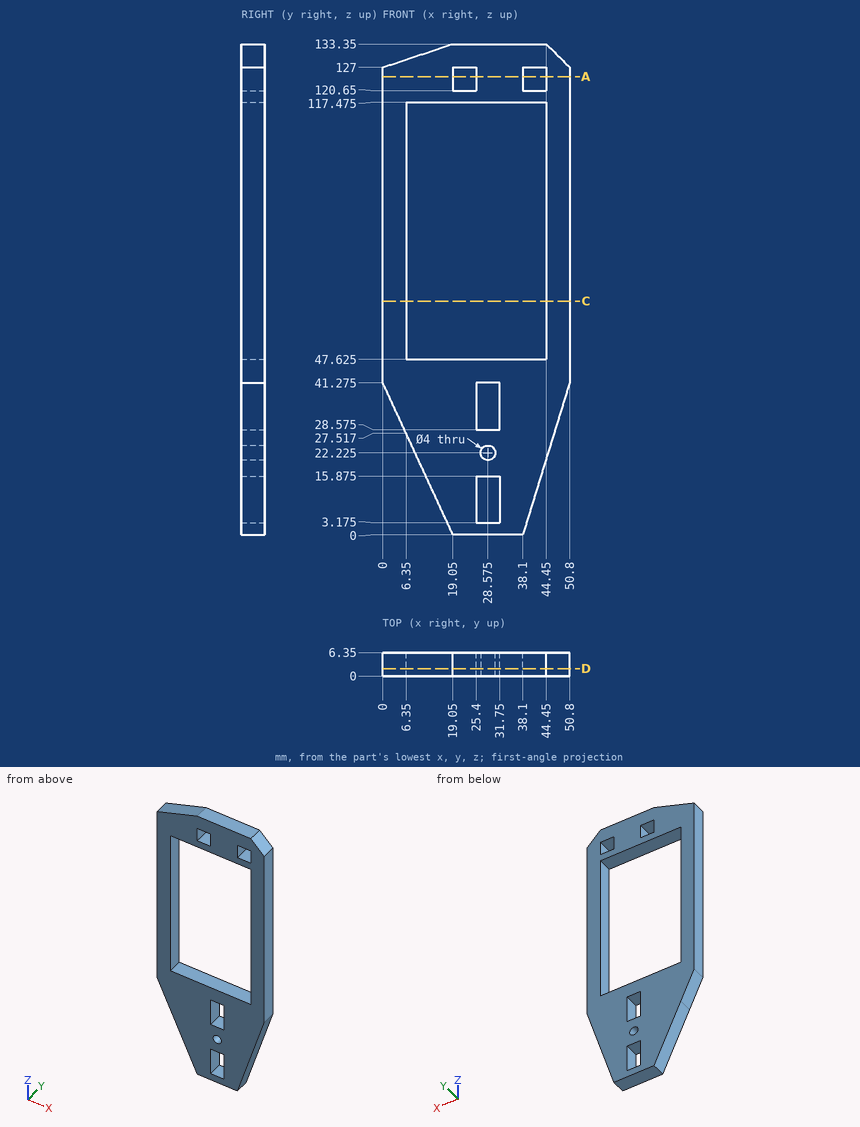
Geometry check sheet. Reference: drawing and pictorial views, mm from the part's lowest x, y, z. Give positions to 0.01 mm unless a question says otherwise; leave off trailing zeros. Order: outer loops, then holes, each group sorted by start corner. A loop starts at its lowest first (then second) coordinate and runs counter-clockwise, first axis right, second up. Notation, with made-up numbers: (44, 18) -> (60, 18) arc R22 cw to (60, 35) -> close; hole circle Ø1 at (88.5, 36). An arc over 180 degrees is marked (long way). Use CSV: the item, a comma, the result in double quotes. Start each with the question number.
1) Sectioned sample at A-A, the plane z = 124.5. Record the boundary of the cut face in (x, y).
2) Sectioned sample at C-C, the plane z = 63.5. Record the boundary of the cut face in (x, y).
3) Go/stop test with flat-tipped pins: P1, Ø3, axis at y = 4, z = 8, coming from the +X side; P2, Ø3, axis at y = 2.5, z = 36, coming from the -X side. Record where each tip stops, or that it passes through.
4) Sectioned sample at D-D, the plane y = 2. Give the number of separate pieces and of enclosed holes in the cut face, plus the area to 3 significant figures.
5) Material ranges on line 1 (X direction, y = 1.25, z = 51.5); line 2 (Z direction, x = 9.5, y = 1.5) (1 decimal); line 3 (Z direction, x = 10, y = 6) (1 decimal), recorded low to high. Write a range as from..to.
Recorded:
1,outline,"(0, 0) -> (19.05, 0) -> (19.05, 6.35) -> (0, 6.35) -> close; (25.4, 0) -> (38.1, 0) -> (38.1, 6.35) -> (25.4, 6.35) -> close; (44.45, 0) -> (50.8, 0) -> (50.8, 6.35) -> (44.45, 6.35) -> close"
2,outline,"(0, 0) -> (6.35, 0) -> (6.35, 6.35) -> (0, 6.35) -> close; (44.45, 0) -> (50.8, 0) -> (50.8, 6.35) -> (44.45, 6.35) -> close"
3,P1,"x = 41.02"
3,P2,"x = 1.74"
4,separate pieces,"1"
4,enclosed holes,"6"
4,area,"3,120 mm2"
5,line 1,"0..6.35, 44.45..50.8"
5,line 2,"20.7..47.6, 117.5..130.2"
5,line 3,"19.6..47.6, 117.5..130.3"
